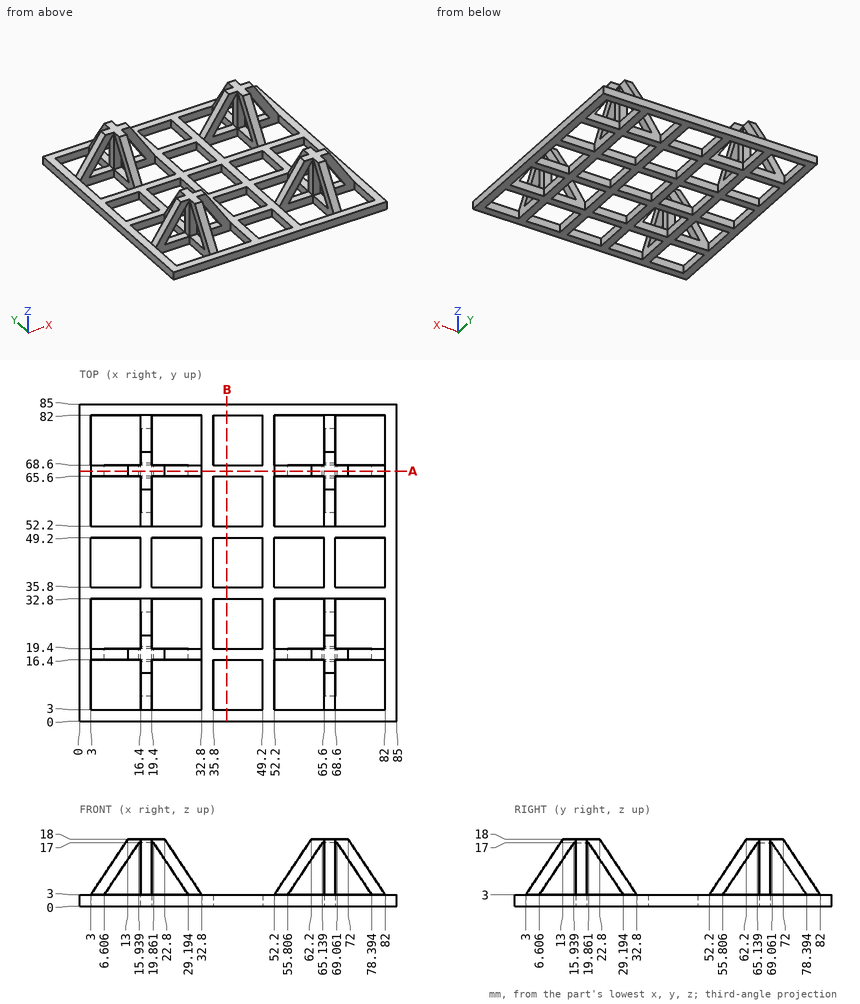
For this review, use the dimensioned drawing (mm, ordinates from the lowest corner) and the shaded views. Give positions to 0.01 mm unless a question says otherwise; leave off trailing zeros. Write each loop counter-clockwise with the first axis right and the second up, starting at its lowest first coordinate (ties: lowest second). Pieces come first, ordered by that corner, then holes.
(1) Consider section A-A, the plane y = 67. Give the number of separate pieces and of enclosed holes in the cut face, and give its area (3 significant figures).
(2) For P1, Ø1, axis at x = 56, y = 30.5, coming from the +Z side; P2, Ø10.5, axis at y = 27, z = 12, coming from the +X side; P3, Ø1.5, axis at x = 59, y = 18.5, coming from the +Z side (1 decimal); P4, Ø3.5, axis at y = 18, z = 9, coming from the +X side, all flat-tipped, find the tip position at first contact; note any pin that passes through.
(3) Consider section B-B, the plane x = 39.5. Give the boundary of the cut face in (y, z).
(4) To check wall thickness, follow L1, parallel to X at y = 8.5, z = 7; L2, parallel to Y at x = 67, z = 5 (1 decimal). State the ranges of each line that lie inside material, in increasing order.
Returned:
1. separate pieces: 1
1. enclosed holes: 4
1. area: 562 mm2
2. P1: passes through
2. P2: stops at x = 68.6
2. P3: stops at z = 14.3
2. P4: stops at x = 79.17
3. outline: (0, 0) - (3, 0) - (3, 3) - (0, 3) - close; (16.4, 0) - (19.4, 0) - (19.4, 3) - (16.4, 3) - close; (32.8, 0) - (35.8, 0) - (35.8, 3) - (32.8, 3) - close; (49.2, 0) - (52.2, 0) - (52.2, 3) - (49.2, 3) - close; (65.6, 0) - (68.6, 0) - (68.6, 3) - (65.6, 3) - close; (82, 0) - (85, 0) - (85, 3) - (82, 3) - close
4. L1: x = 16.4 to 19.4, 65.6 to 68.6
4. L2: y = 4.3 to 7.9, 16.4 to 19.4, 27.9 to 31.5, 53.5 to 57.1, 65.6 to 68.6, 77.1 to 80.7
